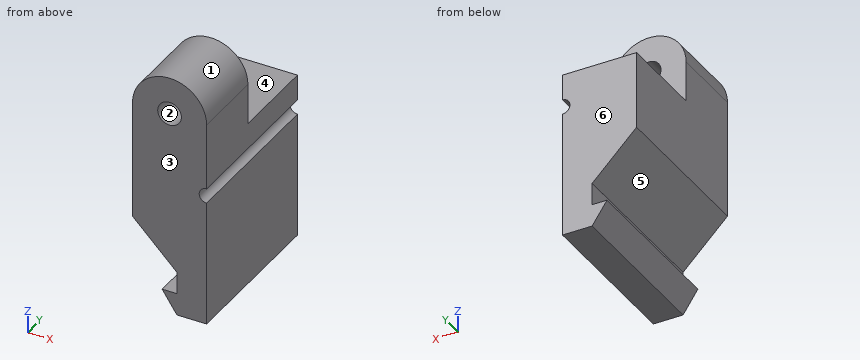
```python
from build123d import *

# Parameters (mm, degrees)
SKETCH1_R           = 1.6
BOSS_EXTRUDE1_DEPTH = 10
BOSS_EXTRUDE2_DEPTH = 12
BOSS_EXTRUDE3_DEPTH = 22
CHAMFER1_SIZE       = 6


with BuildPart() as part:
    # Sketch1 → Boss-Extrude1 (new body)
    with BuildSketch(Plane(origin=(0, 0, 0), x_dir=(1, 0, 0), z_dir=(0, 1, 0))):
        with BuildLine():
            Line((-5, 22), (-5, 0))
            ThreePointArc((-5, 0), (0, -5), (5, 0))
            Line((5, 0), (5, 9))
            ThreePointArc((5, 9), (4, 10), (5, 11))
            Line((5, 11), (5, 22))
            Line((5, 22), (-5, 22))
        make_face()
        with Locations(Location((0, 0, 0), (0, 0, 270))):
            Circle(SKETCH1_R, mode=Mode.SUBTRACT)
    extrude(amount=BOSS_EXTRUDE1_DEPTH)

    # Sketch3 → Boss-Extrude2 (add)
    with BuildSketch(Plane(origin=(0, 10, 0), x_dir=(1, 0, 0), z_dir=(0, 1, 0))):
        with BuildLine():
            Line((5, 5.5), (-5, 5.5))
            Line((-5, 5.5), (-5, 22))
            Line((-5, 22), (5, 22))
            Line((5, 22), (5, 11))
            ThreePointArc((5, 11), (4, 10), (5, 9))
            Line((5, 9), (5, 5.5))
        make_face()
    extrude(amount=BOSS_EXTRUDE2_DEPTH)

    # Sketch5 → Boss-Extrude3 (add)
    with BuildSketch(Plane(origin=(0, 22, 0), x_dir=(1, 0, 0), z_dir=(0, 1, 0))):
        Polygon((5, 22), (5, 28), (1, 28), (-1, 25), (1, 25), (1, 22), align=None)
    extrude(amount=-BOSS_EXTRUDE3_DEPTH)

    # Chamfer1
    chamfer1_edges = [part.edges().sort_by_distance(p)[0] for p in [
        (-5, 11, -22),
    ]]
    chamfer(chamfer1_edges, length=CHAMFER1_SIZE - 0.0001)  # a hair under: the kernel refuses the full size


solid = part.part
```
Model file for the job. Use its own axes, mm. Face numbers are marked on the shaded views. A direction names the side the tool comes from. Coordinates: 2 decimals unless noted, no trailing zeros. Loops run counter-clockwise (first coordinate to the right, second up) from the corner with the lowest first, then second, coordinate; pieces in that order, holes last. Notation, with made-up numbers: (34.5, 84.25) - (84.5, 84.25) arc R18 ccw to (84.5, 116.25) - close; hole circle Ø8 at (-18.75, 62.25). An arc over 180 degrees is marked (long way). Write item = value, one per line. Start each with the question number.
Item 1: Pull direction X, two halves, no side cores. Call the marked faces 1, 2 and 3: +X half, -X half, draft (parallel to the pull), parting line (faces both ways), or undercut.
Item 2: Wall check: probe 1 along Z at (x, y) = (3, 13); probe 2 along Y at (x, z) = (4, 0); probe 3 along Z at (x, y) = (0.5, 15). Give the ranges that are in metal, low to high. Write a range as [from, to].
Item 3: Drop flat-ended pins along their axis: pin 1 Ø1.5 at (x, y) = (-3, 13.5) entering from +Z; pin 2 Ø2.5 at (y, z) = (8, -24) entering from -X; pin 3 Ø2.5 at (x, z) = (0, 0) entering from +Y. Give the stop position or say it passes through.
Item 4: Saw through at D-D, the plane x = 3. List the corners of the cut face in (y, z), then the cut area to 3 significant figures.
Item 5: Saw through at B-B, the plane z = -0.5. List the corners of the cut face in (x, y), then the cut area to 3 significant figures.
Item 6: Saw through at C-C, the plane x = 0. List the corners of the cut face in (y, z), then the cut area to 3 significant figures.
Item 7: 3-axis set-ups, long thin cutter, end or side, ignore diameter. For the marked faces 4, 5 and 6: which of +Z, -Z, +X, -X, +Y, -Y reach the whole face in a straight line?
Answers:
q1.face_1 = parting line
q1.face_2 = undercut
q1.face_3 = draft
q2.probe_1 = [-28, -5.5]
q2.probe_2 = [0, 10]
q2.probe_3 = [-27.25, -25], [-21.5, -5.5]
q3.pin_1 = -5.5
q3.pin_2 = -1
q3.pin_3 = through
q4.outline = (0, -28) - (22, -28) - (22, -5.5) - (10, -5.5) - (10, 4) - (0, 4) - close
q4.area = 590 mm2
q5.outline = (-5, 0) - (-1.52, 0) - (-1.52, 10) - (-5, 10) - close; (1.52, 0) - (5, 0) - (5, 10) - (1.52, 10) - close
q5.area = 69.6 mm2
q6.outline = (0, -26.5) - (22, -26.5) - (22, -25) - (0, -25) - close; (0, -21) - (22, -21) - (22, -5.5) - (10, -5.5) - (10, -1.6) - (0, -1.6) - close; (0, 1.6) - (10, 1.6) - (10, 5) - (0, 5) - close
q6.area = 447 mm2
q7.face_4 = +Z, +X, -X, +Y
q7.face_5 = -X, +Y, -Y
q7.face_6 = +Z, -Z, +X, -X, +Y
